Geometry check sheet. Reference: the model listing, model coordinates, mm. Face numbers are marked on the shaded views. Give positions to 0.01 mm unless a question says otherwise; leave off trailing zeros. Write each loop counter-clockwise with the first axis right and the second up, starting at its lowest first coordinate (ties: lowest second). Pieces come first, ordered by that corner, then holes. Notation, with made-up numbers: (-12.5, 4) - (28.5, 4) arc R19 cw to (28.5, 28) - close; hole circle Ø6 at (25, -16). An arc over 180 degrees is marked (long way). Use a Markdown table: item, result.
```python
from build123d import *

# Parameters (mm, degrees)
SKETCH1_R           = 25
BOSS_EXTRUDE1_DEPTH = 336.383451
SKETCH2_R           = 18.081362876
CUT_EXTRUDE1_DEPTH  = 339.236346519
CHAMFER1_SIZE       = 4.592063
CHAMFER1_SIZE_2     = 7.953686


with BuildPart() as part:
    # Sketch1 → Boss-Extrude1 (new body)
    with BuildSketch(Plane(origin=(0, 0, 0), x_dir=(1, 0, 0), z_dir=(0, 1, 0))):
        with Locations(Location((0, 0, 0), (0, 0, 270))):
            Circle(SKETCH1_R)
    extrude(amount=BOSS_EXTRUDE1_DEPTH)

    # Sketch2 → Cut-Extrude1 (cut, through all)
    with BuildSketch(Plane(origin=(0, 0, 0), x_dir=(1, 0, 0), z_dir=(0, 1, 0))):
        with Locations(Location((0, 0, 0), (0, 0, 270))):
            Circle(SKETCH2_R)
    extrude(amount=CUT_EXTRUDE1_DEPTH, mode=Mode.SUBTRACT)

    # Chamfer1
    # the kernel refuses this chamfer: 7.953686, 4.592063 mm, written as the material it takes off along each edge
    with BuildSketch(Plane(origin=(0, 336.383451, 0), x_dir=(0, 0, 1), z_dir=(-1, 0, 0))) as chamfer1_piece_1:
        Polygon((25, -CHAMFER1_SIZE), (25 - CHAMFER1_SIZE_2, 0), (25, 0), align=None)
    revolve(axis=Axis((0, 336.383451, 0), (0, 1, 0)), mode=Mode.SUBTRACT)
    with BuildSketch(Plane(origin=(0, 0, 0), x_dir=(0, 0, 1), z_dir=(-1, 0, 0))) as chamfer1_piece_2:
        Polygon((25, CHAMFER1_SIZE_2), (25 - CHAMFER1_SIZE, 0), (25, 0), align=None)
    revolve(axis=Axis((0, 0, 0), (0, 1, 0)), mode=Mode.SUBTRACT)


solid = part.part
```
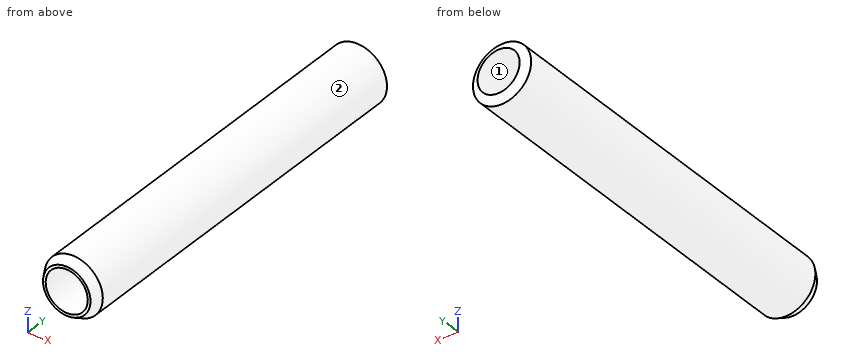
1) Material ranges on L1, parallel to Z at x = 0.5, y = 282.5 (3 decimals); L2, parallel to X at y = 199.5, z = 0; L3, parallel to X at y = 87, z = -1.5, recorded low to high. Write a range as from..to.
Working result:
| item | result |
|---|---|
| L1 | z = -24.995..-18.074, 18.074..24.995 |
| L2 | x = -25..-18.08, 18.08..25 |
| L3 | x = -24.95..-18.02, 18.02..24.95 |
2) Mould release check, pull along X, two halves, no side actions. Record for the marked faces 1 and 2: pulls with the +X half, pulls with the -X half, needs draft (parallel to the pull), parting line crosses it, or undercut.
Working result:
| item | result |
|---|---|
| face 1 | undercut |
| face 2 | parting line crosses it |
3) Section check B-B on x = 0. Record the boundary of the cut face in (y, z).
Working result:
| item | result |
|---|---|
| outline | (0, -20.41) - (7.95, -25) - (331.79, -25) - (335.79, -18.08) - (0, -18.08) - close; (0, 18.08) - (335.79, 18.08) - (331.79, 25) - (7.95, 25) - (0, 20.41) - close |
4) Depth check by flat-ended pin: P1, Ø3, axis at x = 5.5, y = 123, coming from the +Z side; P2, Ø1, axis at y = 216.5, z = -15, coming from the +X side; P3, Ø1, axis at x = -14, y = 37.5, coming from the -Z side; P4, Ø12, axis at x = 17.5, z = -6, coming from the +Y side. Enter the tip coordinate at first touch or a pass-through.
Working result:
| item | result |
|---|---|
| P1 | stops at z = 24.68 |
| P2 | stops at x = 20.37 |
| P3 | stops at z = -21.04 |
| P4 | stops at y = 335.79 |
5) Section check C-C on y = 225.5. Record the boundary of the cut face in (x, z).
Working result:
| item | result |
|---|---|
| outline | circle Ø50 at (0, 0); hole circle Ø36.16 at (0, 0) |
6) Section check A-A on z = 0. Record the boundary of the cut face in (x, y), then the cut area to 3 significant figures.
Working result:
| item | result |
|---|---|
| outline | (-25, 7.95) - (-20.41, 0) - (-18.08, 0) - (-18.08, 335.79) - (-25, 331.79) - close; (18.08, 0) - (20.41, 0) - (25, 7.95) - (25, 331.79) - (18.08, 335.79) - close |
| area | 4,580 mm² |
